Part print with two shaded views. Sizes in mm from the minimum x, y, z corner. Round coordinates to 2 decimals unless told otherwise and drop trailing zeros. Order: outer loops, then holes, each group sorted by start corner. A loop starts at its lowest first (then second) coordinate and runs counter-clockwise, first axis right, second up. Notation, with made-up numbers: (67, -11.75) -> (96, -11.75) arc R21 ccw to (96, 9.25) -> close; hole circle Ø7 at (41.25, 4). An arc over 180 degrees is marked (long way). Use a Markdown table: item, result. Add a question column.
Item 1: Pin check, flat tips, straight feed: pin 1 (4 mm diameter, centred on x = 2, y = 13.5, fed in from -Z); pin 2 (1 mm diameter, centred on y = 11, z = 9, fed in from -X); pin 3 (5.5 mm diameter, centred on x = 116.5, y = 1.5, fed in from +Z); pin 4 (1.5 mm diameter, centred on x = 188.5, y = 7.5, fed in from -Z). Stop position of each tip, or through.
Item 2: Slice it at B-B, the plane x = 121. Give the cut face in (y, z).
Item 3: Probe L1, parallel to X at y = 3.5, z = 12.5; L2, parallel to Z at x = 187.5, y = 7.9; L3, parallel to X at y = 6, z = 6.75. List the from-to ranges inside material, lowest first.
Item 4: Slice it at A-A, the plane y = 13. Give the cut face in (x, z), plus the area to 3 significant figures.
Item 5: Slice it at C-C, the plane z = 2. Give the cut face in (x, y), plus the area to 3 significant figures.
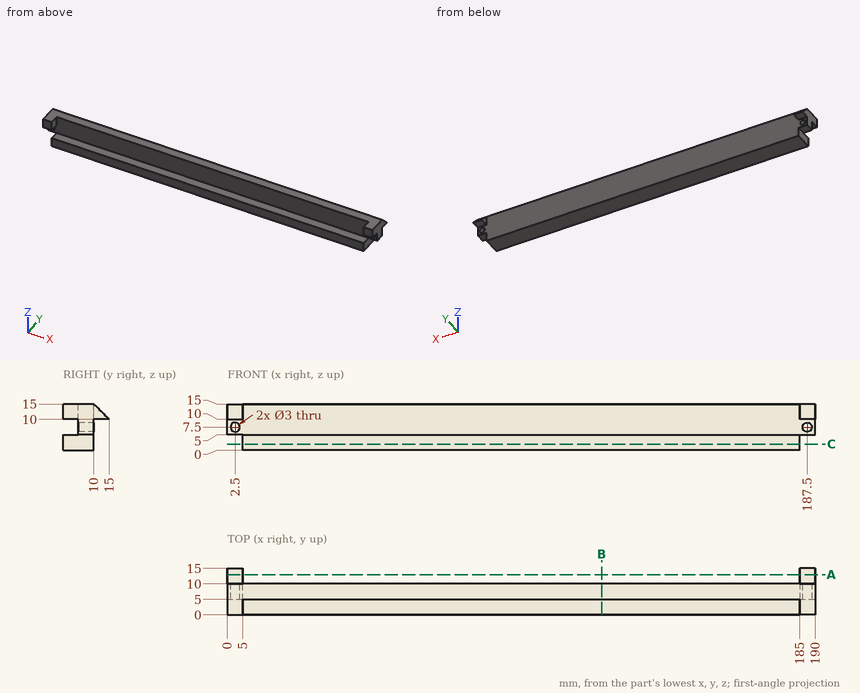
Check sheet entries:
| question | item | result |
|---|---|---|
| 1 | pin 1 | z = 10 |
| 1 | pin 2 | through |
| 1 | pin 3 | z = 5 |
| 1 | pin 4 | z = 5 |
| 2 | outline | (0, 0) -> (10, 0) -> (10, 15) -> (5, 15) -> (5, 5) -> (0, 5) -> close |
| 3 | L1 | 0 to 5, 185 to 190 |
| 3 | L2 | 5 to 6, 9 to 15 |
| 3 | L3 | 0 to 1.2, 3.8 to 186.2, 188.8 to 190 |
| 4 | outline | (0, 10) -> (5, 10) -> (5, 12) -> (0, 12) -> close; (185, 10) -> (190, 10) -> (190, 12) -> (185, 12) -> close |
| 4 | area | 20.0 mm2 |
| 5 | outline | (5, 0) -> (185, 0) -> (185, 10) -> (5, 10) -> close |
| 5 | area | 1,800 mm2 |
